The listing builds one solid part. Answer for the finished solid, in the listing's coordinates (mm). Give positions to 0.01 mm unless a question says otherwise; leave off trailing zeros. Loops run counter-clockwise (first coordinate to the right, second up) from the corner with the lowest first, then second, coordinate; pieces in that order, holes last. Notation, with made-up numbers: (85, 38) - (126, 38) arc R27 cw to (126, 55) - close; hole circle Ø1 at (-34.5, 32.25). An arc over 180 degrees is marked (long way). Write each question's results on one line, items separated by ' | '.
from build123d import *

# Parameters (mm, degrees)
SKETCH1_W                = 53
SKETCH1_H                = 35
BOSS_EXTRUDE1_DEPTH      = 5
FILLET1_R                = 1
SKETCH2_W                = 4.435881082
SKETCH2_H                = 5
BOSS_EXTRUDE2_DEPTH      = 3
BOSS_EXTRUDE2_DEPTH_BACK = 4.5


with BuildPart() as part:
    # Sketch1 → Boss-Extrude1 (new body)
    with BuildSketch(Plane(origin=(0, 0, 0), x_dir=(1, 0, 0), z_dir=(0, 1, 0))):
        Rectangle(SKETCH1_W, SKETCH1_H)
    extrude(amount=BOSS_EXTRUDE1_DEPTH)

    # Fillet1
    fillet1_edges = [part.edges().sort_by_distance(p)[0] for p in [
        (0, 0, 17.5),
        (0, 5, 17.5),
        (0, 0, -17.5),
        (0, 5, -17.5),
    ]]
    fillet(fillet1_edges, radius=FILLET1_R)

    # Sketch2 → Boss-Extrude2 (add, two sides)
    with BuildSketch(Plane.XY.offset(17.5)) as boss_extrude2_sk:
        with Locations((-24.282059459, 2.5)):
            Rectangle(SKETCH2_W, SKETCH2_H)
    extrude(amount=BOSS_EXTRUDE2_DEPTH)
    extrude(boss_extrude2_sk.sketch, amount=-BOSS_EXTRUDE2_DEPTH_BACK)


solid = part.part
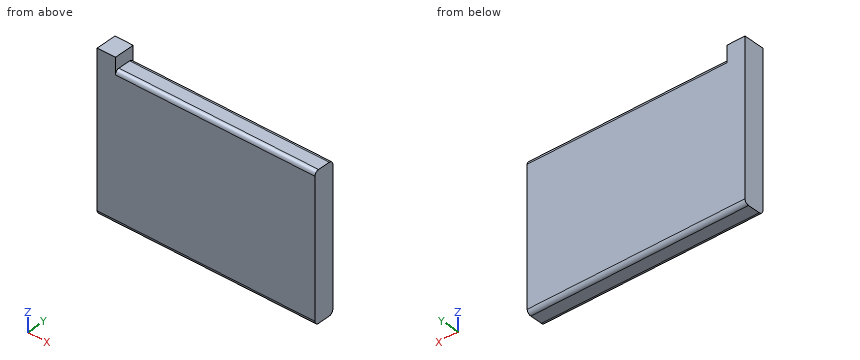
Item 1: A cutting plane is placed at B-B, the plane y = 2.9. Determine the outline of the cut face in (x, z), plus the area to 3 significant figures.
Values found:
outline: (-26.5, -17.5) - (26.5, -17.5) - (26.5, 17.5) - (-22.06, 17.5) - (-22.06, 20.5) - (-26.5, 20.5) - close | area: 1,870 mm²
Item 2: Find the intervals of material crossed by line 1 along Z through (x, y) = (-18.5, 2.95); line 2 along X through (y, z) = (1.2, 18); line 3 along Z through (x, y) = (-24, 0.45), in increasing order. Write a range as [from, to].
Values found:
line 1: z = [-17.5, 17.5] | line 2: x = [-26.5, -22.06] | line 3: z = [-17.34, 20.5]
Item 3: A cutting plane is placed at A-A, the plane x = 15. Determine the outline of the cut face in (y, z).
Values found:
outline: (0, -16.5) arc R1 ccw to (1, -17.5) - (4, -17.5) arc R1 ccw to (5, -16.5) - (5, 16.5) arc R1 ccw to (4, 17.5) - (1, 17.5) arc R1 ccw to (0, 16.5) - close
Item 4: A flat-ended cylindrical pin translates along its axis: P1, Ø0.9, axis at x = 4.5, y = 3, coming from the +Z side. Find the tip coordinate at first contact, or state that the pin passes through.
Values found:
P1: stops at z = 17.5
